from build123d import *

# Parameters (mm, degrees)
F1_DEPTH = 11.938
F3_DEPTH = 9.652
F4_R     = 1.524


with BuildPart() as f1:
    # F0 (on Front) → F1 (new body)
    with BuildSketch(Plane.XZ):
        with BuildLine():
            Line((32.421591, 18.415), (-37.428409, 18.415))
            ThreePointArc((-37.428409, 18.415), (-55.843409, 0), (-37.428409, -18.415))
            Line((-37.428409, -18.415), (32.421591, -18.415))
            ThreePointArc((32.421591, -18.415), (50.836591, 0), (32.421591, 18.415))
        make_face()
    extrude(amount=F1_DEPTH)

    # F2 (on face) → F3 (join)
    with BuildSketch(Plane.XZ.offset(11.938)):
        with BuildLine():
            Line((32.421591, 23.876), (-37.428409, 23.876))
            ThreePointArc((-37.428409, 23.876), (-61.304409, 0), (-37.428409, -23.876))
            Line((-37.428409, -23.876), (32.421591, -23.876))
            ThreePointArc((32.421591, -23.876), (56.297591, 0), (32.421591, 23.876))
        make_face()
    extrude(amount=F3_DEPTH)

    # F4
    f4_edges = [f1.edges().sort_by_distance(p)[0] for p in [
        (-2.503409, -21.59, 23.876),
        (-61.304409, -21.59, 0),
        (-2.503409, -21.59, -23.876),
        (56.297591, -21.59, 0),
        (-2.503409, 0, 18.415),
        (-55.843409, 0, 0),
        (-2.503409, 0, -18.415),
        (50.836591, 0, 0),
    ]]
    fillet(f4_edges, radius=F4_R)


solid = f1.part
Could you check a few things on this model? Use its own coordinates, in mm. A direction names the side the tool comes from. Give positions to 0.01 mm unless a question says otherwise; leave off trailing zeros. Order: outer loops, then holes, each group sorted by start corner. A loop starts at its lowest first (then second) coordinate and runs counter-clockwise, first axis right, second up.
1. Suppose I cut it at C-C (y = -14). Write out the boundary of the cut face in (x, z), plus the area to 3 significant figures.
Answers below:
outline: (-37.43, -23.88) - (32.42, -23.88) arc R23.88 ccw to (32.42, 23.88) - (-37.43, 23.88) arc R23.88 ccw to start
area: 5,130 mm2
2. Which directions (+Z, -Z, +X, -X, +Y, -Y) give clear straight access to the entire face, cutting with the end or side of a thin tool? Please do faces 1 (the cylindrical face through (50.832, -6.658, -0.405)), 2 (the cylindrical face through (-55.84, -6.66, 0.4)), 3 (the flat face through (-3, -7, -18.415)).
Answers below:
face 1: +X, +Y
face 2: -X, +Y
face 3: -Z, +X, -X, +Y
3. Suppose I cut it at D-D (y = -6). Write out the boundary of the cut face in (x, z) (3 decimals).
Answers below:
outline: (-37.428, -18.415) - (32.422, -18.415) arc R18.415 ccw to (32.422, 18.415) - (-37.428, 18.415) arc R18.415 ccw to start
4. Suppose I cut it at A-A (z = 0). Write out the boundary of the cut face in (x, y), plus the area to 3 significant figures.
Answers below:
outline: (-61.3, -20.07) arc R1.52 ccw to (-59.78, -21.59) - (54.77, -21.59) arc R1.52 ccw to (56.3, -20.07) - (56.3, -11.94) - (50.84, -11.94) - (50.84, -1.52) arc R1.52 ccw to (49.31, 0) - (-54.32, 0) arc R1.52 ccw to (-55.84, -1.52) - (-55.84, -11.94) - (-61.3, -11.94) - close
area: 2,410 mm2
5. I need wall thicknesses on L1, parallel to Y at x = 8.5, z = 20; L2, parallel to Z at x = 3.5, y = -7 (3 decimals); L3, parallel to Z at x = 32.5, y = -19. Which ranges of each line are inside material? Lowest first, please.
Answers below:
L1: y = -21.59 to -11.94
L2: z = -18.415 to 18.415
L3: z = -23.88 to 23.88
6. For pin 1 (3 mm diameter, centred on x = -13, y = -7.5, fed in from +Z) (3 decimals); pin 2 (1 mm diameter, centred on y = -5.5, z = 9, fed in from -X); pin 3 (8.5 mm diameter, centred on x = -4.5, y = -5, fed in from -Z) (3 decimals), each with a flat end and sliding along its axis, tell me the tip position at first contact or that it passes through.
Answers below:
pin 1: stops at z = 18.415
pin 2: stops at x = -53.76
pin 3: stops at z = -18.415
7. Suppose I cut it at B-B (x = -31.5). Write out the boundary of the cut face in (y, z) (3 decimals).
Answers below:
outline: (-21.59, -22.352) arc R1.524 ccw to (-20.066, -23.876) - (-11.938, -23.876) - (-11.938, -18.415) - (-1.524, -18.415) arc R1.524 ccw to (0, -16.891) - (0, 16.891) arc R1.524 ccw to (-1.524, 18.415) - (-11.938, 18.415) - (-11.938, 23.876) - (-20.066, 23.876) arc R1.524 ccw to (-21.59, 22.352) - close
